from build123d import *

# Parameters (mm, degrees)
F1_DEPTH = 1.5


with BuildPart() as f1:
    # F0 (on Top) → F1 (new body)
    with BuildSketch(Plane.XY):
        Polygon((45, 65), (0, 0), (55, 0), (55, 65), align=None)
        Polygon((9.542842, 5), (47.619765, 60), (50, 60), (50, 5), align=None, mode=Mode.SUBTRACT)
        Polygon((55, 0), (0, 0), (0, -55), align=None)
        Polygon((5, -42.928932), (5, -5), (42.928932, -5), align=None, mode=Mode.SUBTRACT)
    extrude(amount=F1_DEPTH)


solid = f1.part
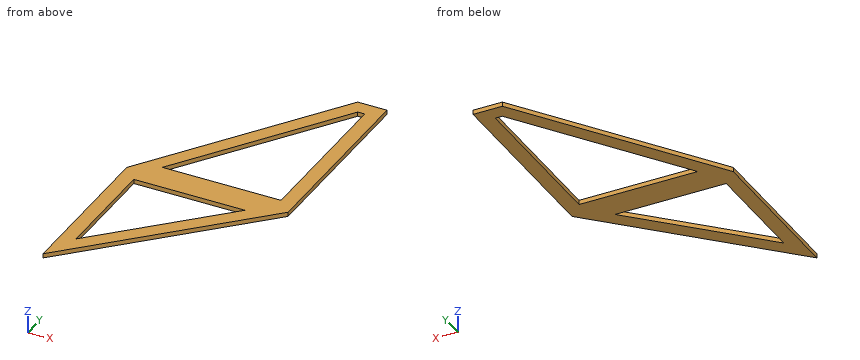
Part model, mm, in its own coordinate system. Round coordinates to 2 decimals unless told otherwise and drop trailing zeros. Write each loop counter-clockwise with the first axis right and the second up, starting at its lowest first coordinate (ties: lowest second). Pieces come first, ordered by that corner, then holes. Notation, with made-up numbers: (-19, -3) - (5, -3) arc R27 cw to (5, 15) - close; hole circle Ø7 at (-21.5, 51). An arc over 180 degrees is marked (long way). Use CSV: the item, a comma, the result in double quotes.
Item 1: Slice it at C-C, the plane x = 22.5. Write the cut outline in (y, z).
Results list:
outline,"(-32.5, 0) - (-25.43, 0) - (-25.43, 1.5) - (-32.5, 1.5) - close; (-5, 0) - (5, 0) - (5, 1.5) - (-5, 1.5) - close; (23.72, 0) - (32.5, 0) - (32.5, 1.5) - (23.72, 1.5) - close"
Item 2: Slice it at B-B, the plane y = 36.5. Write the cut outline in (x, z).
Results list:
outline,"(25.27, 0) - (31.35, 0) - (31.35, 1.5) - (25.27, 1.5) - close; (50, 0) - (55, 0) - (55, 1.5) - (50, 1.5) - close"
Item 3: Slice it at A-A, the plane z = 1.2. Write the cut outline in (x, y), then the cut area to 3 significant figures.
Results list:
outline,"(0, -55) - (55, 0) - (55, 65) - (45, 65) - (0, 0) - close; hole (5, -42.93) - (42.93, -5) - (5, -5) - close; hole (9.54, 5) - (50, 5) - (50, 60) - (47.62, 60) - close"
area,"1,730 mm²"
Item 4: Wall check: L1, parallel to Y at x = 39.5, z = 0.55; L2, parallel to Y at x = 20.5, z = 1.1; L3, parallel to X at y = 23, z = 0.8. Give the ranges that are in metal, low to high.
Results list:
L1,"y = -15.5 to -8.43, -5 to 5, 48.27 to 57.06"
L2,"y = -34.5 to -27.43, -5 to 5, 20.83 to 29.61"
L3,"x = 15.92 to 22, 50 to 55"
Item 5: Slice it at D-D, the plane x = 46.5. Write the cut outline in (y, z), then the cut area to 3 significant figures.
Results list:
outline,"(-8.5, 0) - (5, 0) - (5, 1.5) - (-8.5, 1.5) - close; (58.38, 0) - (65, 0) - (65, 1.5) - (58.38, 1.5) - close"
area,"30.2 mm²"
